from build123d import *

# Parameters (mm, degrees)
ESQUISSE1_W             = 180
ESQUISSE1_H             = 180
BOSS_EXTRU_1_DEPTH      = 96
CONG_1_R                = 32
ESQUISSE2_R             = 20
ESQUISSE2_R_2           = 5
ENL_V_MAT_EXTRU_1_DEPTH = 9.6


with BuildPart() as part:
    # Esquisse1 → Boss.-Extru.1 (new body)
    with BuildSketch(Plane.XY):
        Rectangle(ESQUISSE1_W, ESQUISSE1_H)
    extrude(amount=BOSS_EXTRU_1_DEPTH)

    # Congé1
    cong_1_edges = [part.edges().sort_by_distance(p)[0] for p in [
        (90, -90, 48),
        (-90, -90, 48),
        (-90, 90, 48),
        (90, 90, 48),
    ]]
    fillet(cong_1_edges, radius=CONG_1_R)

    # Esquisse2 → Enlèv. mat.-Extru.1 (cut)
    with BuildSketch(Plane.XY.offset(96)):
        with Locations((54, 54)):
            Circle(ESQUISSE2_R)
        with Locations((54, -54)):
            Circle(ESQUISSE2_R)
        with Locations((-45, 0)):
            Circle(ESQUISSE2_R_2)
    extrude(amount=-ENL_V_MAT_EXTRU_1_DEPTH, mode=Mode.SUBTRACT)


solid = part.part
Part model, mm, in its own coordinate system. A direction names the side the tool comes from. Round coordinates to 2 decimals unless told otherwise and drop trailing zeros. Write each loop counter-clockwise with the first axis right and the second up, starting at its lowest first coordinate (ties: lowest second). Pieces come first, ordered by that corner, then holes. Notation, with made-up numbers: M -27.5,-17 L -9.5,-17 A9 ccw -9.5,-2 Z; hole C 14,-25 d11. An arc over 180 degrees is marked long. Return JSON: item names as keys, results as strings. Group by question number.
(1) Saw through at C-C on x = 42. Write the cut outline in (y, z), then the cut area to 3 significant figures.
(2) Saw through at D-D on x = -69. Write the cut outline in (y, z).
(3) Drill centre lines: probe 1 along Y at (x, z) = (54, 91); probe 2 along Y at (x, z) = (-45, 90.25); probe 3 along Z at (x, y) = (43.5, -55). Where is each one in solid material? Low to high.
(4) Two-plate mould, pull along X, no slides. Class faces 3 (the face through (90, -1, 47)), 4 (the face through (-90, -1, 47)), 5 (the face through (73.076, -47.993, 91.267)): +X half, -X half, draft (parallel to the pull), parting line (faces both ways), or undercut.
(5) Which spindle directions (+Z, -Z, +X, -X, +Y, -Y) get a long thin tool onto all of the face, cutting with end or side? Do faces 1 (the face through (73.076, 60.007, 91.267)), 2 (the face through (-1, -90, 47)). Say none if no direction does.
(6) Saw through at A-A on y = 54. Write the cut outline in (x, z), then the cut area to 3 significant figures.
(7) Pin check, flat tips, straight feed: pin 1 Ø9 at (x, y) = (-45, 0) entering from +Z; pin 2 Ø10 at (y, z) = (-64, 46.5) entering from +X. Stop position of each tip, or through.
(8) Saw through at B-B on z = 12. Write the cut outline in (x, y).
Returned:
{
 "1": {"outline": "M -90,0 L 90,0 L 90,96 L 70,96 L 70,86.4 L 38,86.4 L 38,96 L -38,96 L -38,86.4 L -70,86.4 L -70,96 L -90,96 Z", "area": "16,700 mm²"},
 "2": {"outline": "M -88.05,0 L 88.05,0 L 88.05,96 L -88.05,96 Z"},
 "3": {"probe 1": "-90 to -74, -34 to 34, 74 to 90", "probe 2": "-90 to -5, 5 to 90", "probe 3": "0 to 86.4"},
 "4": {"face 3": "+X half", "face 4": "-X half", "face 5": "undercut"},
 "5": {"face 1": "+Z", "face 2": "+Z, -Z, +X, -X, -Y"},
 "6": {"outline": "M -90,0 L 90,0 L 90,96 L 74,96 L 74,86.4 L 34,86.4 L 34,96 L -90,96 Z", "area": "16,900 mm²"},
 "7": {"pin 1": "z = 86.4", "pin 2": "x = 89.98"},
 "8": {"outline": "M -90,-58 A32 ccw -58,-90 L 58,-90 A32 ccw 90,-58 L 90,58 A32 ccw 58,90 L -58,90 A32 ccw -90,58 Z"}
}
